For this review, take the finished solid that the model builds, in its own axes (mm). A direction names the side the tool comes from. Give positions to 0.01 mm unless a question says otherwise; leave off trailing zeros. Write each loop counter-clockwise with the first axis right and the second up, starting at its lowest first coordinate (ties: lowest second). Pieces come first, ordered by that corner, then holes. Notation, with made-up numbers: M 29.5,20 L 54.5,20 A18 cw 54.5,39 Z; hole C -4.75,63 d9. An arc over 180 degrees is marked long. Write item = value, one per line.
```python
from build123d import *

# Parameters (mm, degrees)
BOSS_EXTRU_1_DEPTH      = 15
CONG_1_R                = 8
ESQUISSE2_R             = 2.5
ENL_V_MAT_EXTRU_1_DEPTH = 15


with BuildPart() as part:
    # Esquisse1 → Boss.-Extru.1 (new body)
    with BuildSketch(Plane(origin=(0, 0, 0), x_dir=(1, 0, 0), z_dir=(0, 1, 0))):
        Polygon((15, -8.660254038), (10, 0), (5, -8.660254038), (0, -5.773502692), (0, -100), (20, -100), (20, -5.773502692), align=None)
        with BuildLine():
            Line((5, 8.660254038), (10, 11.547005384))
            Line((10, 11.547005384), (-64.674337148, 54.660254038))
            ThreePointArc((-64.674337148, 54.660254038), (-70.744889509, 55.459457418), (-75.602540378, 51.732050808))
            Line((-75.602540378, 51.732050808), (-77.602540378, 48.267949192))
            ThreePointArc((-77.602540378, 48.267949192), (-78.401743758, 42.197396832), (-74.674337148, 37.339745962))
            Line((-74.674337148, 37.339745962), (0, -5.773502692))
            Line((0, -5.773502692), (0, 0))
            Line((0, 0), (10, 0))
            Line((10, 0), (5, 8.660254038))
        make_face()
        with BuildLine():
            Line((10, 11.547005384), (15, 8.660254038))
            Line((15, 8.660254038), (10, 0))
            Line((10, 0), (20, 0))
            Line((20, 0), (20, -5.773502692))
            Line((20, -5.773502692), (94.674337148, 37.339745962))
            ThreePointArc((94.674337148, 37.339745962), (98.401743758, 42.197396832), (97.602540378, 48.267949192))
            Line((97.602540378, 48.267949192), (95.602540378, 51.732050808))
            ThreePointArc((95.602540378, 51.732050808), (90.744889509, 55.459457418), (84.674337148, 54.660254038))
            Line((84.674337148, 54.660254038), (10, 11.547005384))
        make_face()
        Polygon((10, 0), (15, 8.660254038), (10, 11.547005384), (5, 8.660254038), align=None)
        Polygon((20, 0), (10, 0), (15, -8.660254038), (20, -5.773502692), align=None)
        Polygon((5, -8.660254038), (10, 0), (0, 0), (0, -5.773502692), align=None)
    extrude(amount=BOSS_EXTRU_1_DEPTH)

    # Cong_1
    cong_1_edges = [part.edges().sort_by_distance(p)[0] for p in [
        (20, 7.5, 100),
        (0, 7.5, 100),
    ]]
    fillet(cong_1_edges, radius=CONG_1_R)

    # Esquisse2 → Enl_v. mat.-Extru.1 (cut)
    with BuildSketch(Plane(origin=(0, 15, 0), x_dir=(1, 0, 0), z_dir=(0, 1, 0))):
        with Locations(Location((10, 0, 0), (0, 0, 270))):
            Circle(ESQUISSE2_R)
    extrude(amount=-ENL_V_MAT_EXTRU_1_DEPTH, mode=Mode.SUBTRACT)


solid = part.part
```
1. We need section C-C, the plane z = 79. Write out the cut boundary in (x, y).
Responses:
outline = M 0,0 L 20,0 L 20,15 L 0,15 Z
2. The part is to be moulded in two halves that separate along X. For faces 1 (the face through (20, 7, 49)), 2 (the face through (10, 15, 4)), 3 (the face through (-26.81, 7.4, -32.8)), say which applies: +X half, -X half, draft (parallel to the pull), parting line (faces both ways), or undercut.
Responses:
face_1 = +X half
face_2 = draft
face_3 = undercut
3. For line 1 along X through (y, z) = (11.75, 40.5); line 2 along X through (y, z) = (14, -17); line 3 along Z through (x, y) = (11, 11.5), list the stretches that pass through material, from the lowest coordinate up. Write a range as from..to.
Responses:
line_1 = 0..20
line_2 = -39.44..0.56, 19.44..59.44
line_3 = -12.12..-2.29, 2.29..100
4. We need section D-D, the plane x = 18. Write out the cut boundary in (y, z), then the cut area to 3 significant figures.
Responses:
outline = M 0,-16.17 L 15,-16.17 L 15,97.29 L 0,97.29 Z
area = 1,700 mm2
5. Machinability: for faces 4 (the face through (98.379, 7.395, -42.113)), 5 (the face through (0, 7, 48)), 6 (the face through (47.86, 7.395, -33.405)), which of the approach directions +Z, -Z, +X, -X, +Y, -Y give a long, thin tool a straight path to every point of the face, cutting with its end or side? Answer none if there is none.
Responses:
face_4 = +X, +Y, -Y
face_5 = +Z, -X, +Y, -Y
face_6 = -Z, +Y, -Y
6. We need section A-A, the plane y = 5.25. Write out the cut boundary in (x, z), then the cut area to 3 significant figures.
Responses:
outline = M -77.6,-48.27 L -75.6,-51.73 A8 ccw -64.67,-54.66 L 10,-11.55 L 84.67,-54.66 A8 ccw 95.6,-51.73 L 97.6,-48.27 A8 ccw 94.67,-37.34 L 20,5.77 L 20,92 A8 ccw 12,100 L 8,100 A8 ccw 0,92 L 0,5.77 L -74.67,-37.34 A8 ccw Z; hole C 10,0 d5
area = 5,720 mm2
7. Insertion check: P1, Ø8, axis at y = 5, z = 64.5, coming from the +X side; P2, Ø7.5, axis at y = 11, z = 51, coming from the -X side. Each pin has a flat end and moves straight along its axis. Give the tip position at first contact, or say it passes through.
Responses:
P1 = 20
P2 = 0
8. We need section B-B, the plane z = 0. Write out the cut boundary in (x, y), then the cut area to 3 significant figures.
Responses:
outline = M -10,0 L 7.5,0 L 7.5,15 L -10,15 Z; M 12.5,0 L 30,0 L 30,15 L 12.5,15 Z
area = 525 mm2
